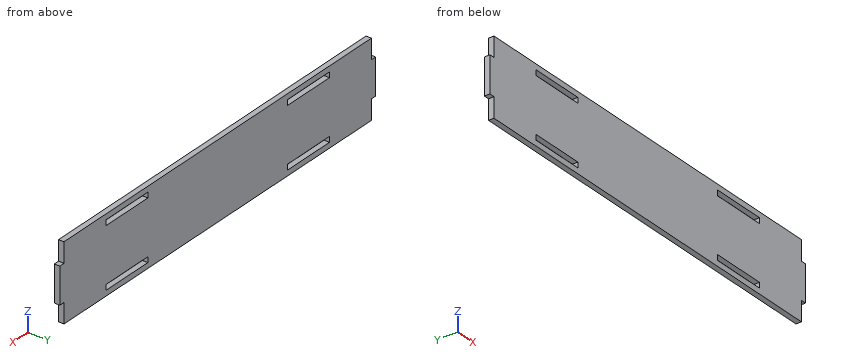
from build123d import *

# Parameters (mm, degrees)
SKETCH1_W           = 30
SKETCH1_H           = 3
BOSS_EXTRUDE1_DEPTH = 3


with BuildPart() as part:
    # Sketch1 → Boss-Extrude1 (new body)
    with BuildSketch(Plane(origin=(0, 0, 0), x_dir=(1, 0, 0), z_dir=(0, 1, 0))):
        Polygon((0, 0), (220, 0), (220, 11), (223, 11), (223, 31), (220, 31), (220, 42), (0, 42), (0, 31), (-3, 31), (-3, 11), (0, 11), align=None)
        with Locations((45, 37.5)):
            Rectangle(SKETCH1_W, SKETCH1_H, mode=Mode.SUBTRACT)
        with Locations((175, 37.5)):
            Rectangle(SKETCH1_W, SKETCH1_H, mode=Mode.SUBTRACT)
        with Locations((175, 4.5)):
            Rectangle(SKETCH1_W, SKETCH1_H, mode=Mode.SUBTRACT)
        with Locations((45, 4.5)):
            Rectangle(SKETCH1_W, SKETCH1_H, mode=Mode.SUBTRACT)
    extrude(amount=BOSS_EXTRUDE1_DEPTH)


solid = part.part
Model file for the job. Use its own axes, mm. Round coordinates to 2 decimals unless told otherwise and drop trailing zeros. Order: outer loops, then holes, each group sorted by start corner. A loop starts at its lowest first (then second) coordinate and runs counter-clockwise, first axis right, second up.
(1) Pin check, flat tips, straight feed: pin 1 (0.9 mm diameter, centred on y = 1.5, z = -7, fed in from +X); pin 2 (0.9 mm diameter, centred on y = 2, z = -37.5, fed in from -X); pin 3 (0.9 mm diameter, centred on x = -1, y = 1, fed in from +Z). Stop position of each tip, or through.
(2) Band-saw the part on A-A (x = 51.5). List the corners of the cut face in (y, z).
(3) Drill centre lines: line 1 (Z direction, x = 49, y = 2.75); line 2 (X direction, y = 0.95, z = -37.5); line 3 (X direction, y = 1.35, z = -7.5). Where is each one in solid material? Low to high.
(4) Band-saw the part on B-B (y = 1.25). List the corners of the cut face in (x, z).
Verdict:
1. pin 1: stops at x = 220
1. pin 2: stops at x = 0
1. pin 3: stops at z = -11
2. outline: (0, -42) - (3, -42) - (3, -39) - (0, -39) - close; (0, -36) - (3, -36) - (3, -6) - (0, -6) - close; (0, -3) - (3, -3) - (3, 0) - (0, 0) - close
3. line 1: z = -42 to -39, -36 to -6, -3 to 0
3. line 2: x = 0 to 30, 60 to 160, 190 to 220
3. line 3: x = 0 to 220
4. outline: (-3, -31) - (0, -31) - (0, -42) - (220, -42) - (220, -31) - (223, -31) - (223, -11) - (220, -11) - (220, 0) - (0, 0) - (0, -11) - (-3, -11) - close; hole (30, -39) - (60, -39) - (60, -36) - (30, -36) - close; hole (30, -6) - (60, -6) - (60, -3) - (30, -3) - close; hole (160, -39) - (190, -39) - (190, -36) - (160, -36) - close; hole (160, -6) - (190, -6) - (190, -3) - (160, -3) - close
